from build123d import *

# Parameters (mm, degrees)
SKETCH1_R           = 1.5
SKETCH1_R_2         = 4
SKETCH1_W           = 5.2
SKETCH1_H           = 13.2
BOSS_EXTRUDE1_DEPTH = 5


with BuildPart() as part:
    # Sketch1 → Boss-Extrude1 (new body)
    with BuildSketch(Plane.XY):
        with BuildLine():
            Line((-139.3729909, 139.350971349), (50.6270091, 139.350971349))
            ThreePointArc((50.6270091, 139.350971349), (54.162543006, 137.886505255), (55.6270091, 134.350971349))
            Line((55.6270091, 134.350971349), (55.6270091, 84.350971349))
            ThreePointArc((55.6270091, 84.350971349), (54.162543006, 80.815437443), (50.6270091, 79.350971349))
            Line((50.6270091, 79.350971349), (-139.3729909, 79.350971349))
            ThreePointArc((-139.3729909, 79.350971349), (-142.908524806, 80.815437443), (-144.3729909, 84.350971349))
            Line((-144.3729909, 84.350971349), (-144.3729909, 134.350971349))
            ThreePointArc((-144.3729909, 134.350971349), (-142.908524806, 137.886505255), (-139.3729909, 139.350971349))
        make_face()
        with Locations((48.024043129, 109.750971349)):
            Circle(SKETCH1_R, mode=Mode.SUBTRACT)
        with Locations(Location((-136.770024929, 109.350971349, 0), (0, 0, 180))):
            Circle(SKETCH1_R, mode=Mode.SUBTRACT)
        with Locations((-44.3729909, 109.750971349)):
            Circle(SKETCH1_R_2, mode=Mode.SUBTRACT)
        with Locations((-17.9729909, 109.750971349)):
            Circle(SKETCH1_R_2, mode=Mode.SUBTRACT)
        with Locations((-136.770024929, 125.150971349)):
            Rectangle(SKETCH1_W, SKETCH1_H, mode=Mode.SUBTRACT)
        with Locations((48.024043129, 93.950971349)):
            Rectangle(SKETCH1_W, SKETCH1_H, mode=Mode.SUBTRACT)
        with Locations((48.024043129, 125.550971349)):
            Rectangle(SKETCH1_W, SKETCH1_H, mode=Mode.SUBTRACT)
        with Locations((-136.770024929, 93.550971349)):
            Rectangle(SKETCH1_W, SKETCH1_H, mode=Mode.SUBTRACT)
    extrude(amount=BOSS_EXTRUDE1_DEPTH)


solid = part.part
Could you check a few things on this model? Use its own coordinates, in mm. A direction names the side the tool comes from. Give positions to 0.01 mm unless a question says otherwise; leave off trailing zeros. Loops run counter-clockwise (first coordinate to the right, second up) from the corner with the lowest first, then second, coordinate; pieces in that order, holes last. Notation, with made-up numbers: (6.5, 29) -> (45.5, 29) arc R7 cw to (45.5, 39) -> close; hole circle Ø6 at (63.5, 49). An arc over 180 degrees is marked (long way). Answer as CSV lines item,"result". Start each with the question number.
(1) We'd pull the mould along Y, two halves only. Please class faces 1 (the cylindrical face through (-16.13, 106.2, 2.46)), 2 (the flat face through (-43, 116, 0)), 3 (the cylindrical face through (-142.947, 137.847, 2.465)), 4 (the flat face through (50.624, 125, 2)): released by +Y, released by -Y, zero draft, split by the parting line, or undercut.
(2) If we section it at B-B on z = 1.3: Count the separate pieces of the cut face and the enclosed holes in it, then the cut area to 3 significant figures.
(3) I need wall thicknesses on probe 1 along X at (y, z) = (90, 2.2); probe 2 along X at (y, z) = (109.5, 4.35); probe 3 along X at (y, z) = (87, 0.45). Which ranges of each line are inside material? Lowest first, please.
(4) Which directions (+Z, -Z, +X, -X, +Y, -Y) give clear straight access to the entire face, cutting with the end or side of a thin tool? Please do faces 5 (the flat face through (48, 87.351, 2)), 6 (the cylindrical face through (54.12, 137.93, 2.46)).
(5) If we section it at A-A on y = 127.5: Write out the boundary of the cut face in (x, z), then the cut area to 3 significant figures.
Computed:
1,face 1,"undercut"
1,face 2,"zero draft"
1,face 3,"released by +Y"
1,face 4,"undercut"
2,separate pieces,"1"
2,enclosed holes,"8"
2,area,"11,600 mm2"
3,probe 1,"x = -144.37 to -139.37, -134.17 to 45.42, 50.62 to 55.63"
3,probe 2,"x = -144.37 to -138.26, -135.28 to -48.37, -40.38 to -21.97, -13.98 to 46.55, 49.5 to 55.63"
3,probe 3,"x = -144.37 to -139.37, -134.17 to 55.63"
4,face 5,"+Z, -Z"
4,face 6,"+Z, -Z, +X, +Y"
5,outline,"(-144.37, 0) -> (-139.37, 0) -> (-139.37, 5) -> (-144.37, 5) -> close; (-134.17, 0) -> (45.42, 0) -> (45.42, 5) -> (-134.17, 5) -> close; (50.62, 0) -> (55.63, 0) -> (55.63, 5) -> (50.62, 5) -> close"
5,area,"948 mm2"
